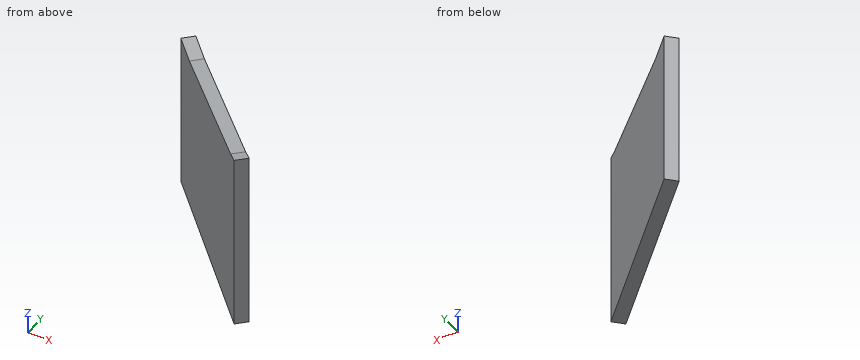
Autodesk Inventor part; units mm, degrees
ref_plane "YZ Plane" through (0, 0, 0) normal (1, 0, 0) x (0, 1, 0)
ref_plane "XZ Plane" through (0, 0, 0) normal (0, 1, 0) x (-1, 0, 0)
ref_plane "XY Plane" through (0, 0, 0) normal (0, 0, 1) x (1, 0, 0)
sketch "Esboço1" plane through (0, 0, 0) normal (0, 0, 1) x (1, 0, 0)
  line L0 (-71, -40) -> (-71, -37)
  line L1 (-71, -37) -> (-38.1386, -69.8614)
  line L2 (14.6, -69.1) -> (-41.9, -69.1)
  line L3 (-38.9, -69.1) -> (-71, -37)
  line L4 (-71, -37) -> (-73.1213, -39.1213)
  line L5 (-73.1213, -39.1213) -> (-41.0213, -71.2213)
  line L6 (-41.0213, -71.2213) -> (-38.9, -69.1)
  point P0 (0, 0)
  dimension "d0" = 3
  dimension "d1" = 45
  dimension "d2" = 3
extrude "Extrusão1" add sketch "Esboço1" against normal blind 11.5
sketch "Esboço3" plane through (0, 0, 0) normal (0, 0, 1) x (1, 0, 0)
  line L0 (-38.9, -69.1) -> (-41.0213, -71.2213)
  line L1 (-38.9, -69.1) -> (-71, -37)
  line L2 (-71, -37) -> (-73.1213, -39.1213)
  line L3 (-73.1213, -39.1213) -> (-41.0213, -71.2213)
  line L4 (-41.0213, -71.2213) -> (-38.9, -69.1)
  point P0 (0, 0)
extrude "Extrusão2" add sketch "Esboço3" along normal blind 35.6
sketch "Esboço6" plane through (-73.1213, -39.1213, 35.6) normal (-0.7071, -0.7071, 0) x (-0.7071, 0.7071, 0)
  line L0 (-42.3963, 7.117) -> (-7.2426, 11.5)
  line L1 (55.3259, 11.5) -> (-7.2426, 11.5)
  line L2 (-42.3963, 7.117) -> (-83.2265, -3.0646)
  line L3 (-45.3963, 0) -> (0, 0)
  line L4 (-45.3963, 47.1) -> (-45.3963, 0)
  line L5 (0, 0) -> (-45.3963, 0)
  line L6 (-45.3963, 0) -> (-45.3963, 14)
  line L7 (-45.3963, 14) -> (0, 14)
  line L8 (0, 14) -> (0, 0)
  point P0 (-24.0416, 35.6)
  point P1 (-45.3963, 6.3689)
  point P2 (0, 11.5)
extrude "Extrusão3" cut sketch "Esboço6" against normal blind 19 contours L0 L1 L8 L3 L4 L2
properties part number "diagonal"
Source: CAD feature listing. Evaluate the final solid. Frame: model axes, mm. Coordinates: 2 decimals unless noted, no trailing zeros. Write each loop counter-clockwise with the first axis right and the second up, starting at its lowest first coordinate (ties: lowest second). Pieces come first, ordered by that corner, then holes. Notation, with made-up numbers: (7.5, 0) -> (49.5, 0) arc R31 cw to (49.5, 33) -> close; hole circle Ø11 at (-39.75, 71.5). An arc over 180 degrees is marked (long way). Return JSON: item names as keys, results as strings. Group by question number.
1) Section query A-A, the plane x = -42. Return loops of the section in (y, z), plus the area to 3 significant figures.
2) Section query B-B, the plane z = -8.5. Return loops of the section in (x, y), plus the area to 3 significant figures.
3) Ray query, line 1 along Z through (x, y) = (-53, -57); line 2 along X through (y, z) = (-52.5, -7.5); line 3 along Y through (x, z) = (-57.5, 20.5). Return the intervals inside material, ascending.
4) Contact query for flat-ended pins moving along their axis: P1, Ø10, axis at y = -55, z = 1.5, coming from the +X side; P2, Ø2, axis at x = -70.5, y = -40.5, coming from the +Z side; P3, Ø4, axis at y = -50.5, z = 10, coming from the -X side; P4, Ø10, axis at x = -52, y = -47, coming from the -Z side. Output: stop coordinate, or through.
5) Section query D-D, the plane x = -67. Return loops of the section in (y, z), plus the area to 3 significant figures.
6) Section query C-C, the plane y = -57.5. Return loops of the section in (x, z).
From the geometry:
{
 "1": {"outline": "(-70.24, -11.5) -> (-66, -11.5) -> (-66, 28.31) -> (-67.96, 28.48) -> (-70.24, 28.89) -> close", "area": "170 mm²"},
 "2": {"outline": "(-73.12, -39.12) -> (-41.02, -71.22) -> (-38.9, -69.1) -> (-71, -37) -> close", "area": "136 mm²"},
 "3": {"line 1": "-11.5 to 26.55", "line 2": "-59.74 to -55.5", "line 3": "-54.74 to -50.5"},
 "4": {"P1": "x = -48", "P2": "z = 24.1", "P3": "x = -63.74", "P4": "through"},
 "5": {"outline": "(-45.24, -11.5) -> (-41, -11.5) -> (-41, 24.1) -> (-43.24, 24.1) -> (-45.24, 24.28) -> close", "area": "151 mm²"},
 "6": {"outline": "(-54.74, -11.5) -> (-50.5, -11.5) -> (-50.5, 26.81) -> (-54.74, 26.44) -> close"}
}
